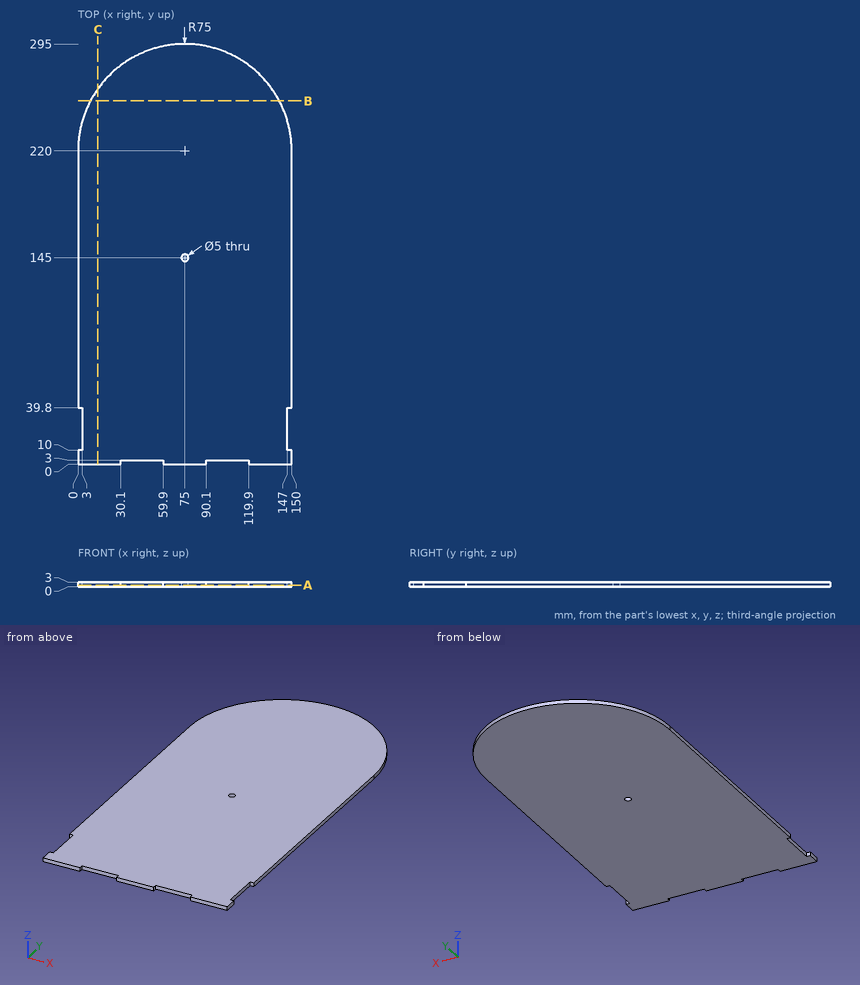
Input: dimensioned drawing with shaded views. Units: mm. Origin: part minimum x, y, z. Coordinates: 2 decimals unless noted, no trailing zeros. Order: outer loops, then holes, each group sorted by start corner. A loop starts at its lowest first (then second) coordinate and runs counter-clockwise, first axis right, second up. Notation, with made-up numbers: (72.5, -40) - (97.5, -40) arc R13 cw to (97.5, -23) - close; hole circle Ø3 at (-9.5, 70.5). An arc over 180 degrees is marked (long way). Return JSON: item names as keys, results as strings. Group by question number.
1. Cut plane B-B (y = 255). Output: boundary loops of the cut face in (x, z), plus the area to 3 significant figures.
2. Material intervals for line 1 along Y through (x, z) = (75, 2.1); line 2 along X through (y, z) = (145, 1); line 3 along X through (y, z) = (38.5, 0.25), sorted ascending. Write a range as [from, to].
3. Cut plane A-A (z = 0.95). Output: boundary loops of the cut face in (x, y).
4. Cut plane C-C (x = 14). Output: boundary loops of the cut face in (y, z).
5. Pin query (flat end, axial travel): pin 1 (1.5 mm diameter, centred on y = 19.5, z = 2, fed in from +X); pin 2 (1 mm diameter, centred on y = 251.5, z = 0.5, fed in from +X); pin 3 (1.5 mm diameter, centred on x = 23.5, z = 1.5, fed in from +Y). Return the tip coordinate at first contact, or that it passes through.
Resolved:
{
 "1": {"outline": "(8.67, 0) - (141.33, 0) - (141.33, 3) - (8.67, 3) - close", "area": "398 mm²"},
 "2": {"line 1": "y = [0, 142.5], [147.5, 295]", "line 2": "x = [0, 72.5], [77.5, 150]", "line 3": "x = [3, 147]"},
 "3": {"outline": "(0, 0) - (30.1, 0) - (30.1, 3) - (59.9, 3) - (59.9, 0) - (90.1, 0) - (90.1, 3) - (119.9, 3) - (119.9, 0) - (150, 0) - (150, 10) - (147, 10) - (147, 39.8) - (150, 39.8) - (150, 220) arc R75 ccw to (0, 220) - (0, 39.8) - (3, 39.8) - (3, 10) - (0, 10) - close; hole circle Ø5 at (75, 145)"},
 "4": {"outline": "(0, 0) - (263.63, 0) - (263.63, 3) - (0, 3) - close"},
 "5": {"pin 1": "stops at x = 147", "pin 2": "stops at x = 143.29", "pin 3": "stops at y = 275.22"}
}
